Work out the finished part from the listing and answer in its coordinate system (mm). Face numbers are marked on the shaded views. A direction names the side the tool comes from. Round coordinates to 2 decimals unless told otherwise and drop trailing zeros. Order: outer loops, then holes, each group sorted by start corner. A loop starts at its lowest first (then second) coordinate and runs counter-clockwise, first axis right, second up. Notation, with made-up numbers: (80.25, 61) - (134.25, 61) arc R13 cw to (134.25, 81) - close; hole circle Ø9 at (87.25, 17.5). An arc over 180 degrees is marked (long way). One line per question, with ' | ' between items. Start each with the question number.
from build123d import *

# Parameters (mm, degrees)
BOSS_EXTRUDE1_DEPTH = 15.875
BOSS_EXTRUDE2_DEPTH = 3.175
CUT_EXTRUDE1_REACH  = 24.393
FILLET2_R           = 1.778
FILLET3_R           = 1.778


with BuildPart() as part:
    # Sketch1 → Boss-Extrude1 (new body)
    with BuildSketch(Plane(origin=(0, 0, 0), x_dir=(0, 0, -1), z_dir=(1, 0, 0))):
        Polygon((0, 0), (-1.016, 0), (-1.016, 10.541), (13.97, 10.541), (13.97, 0), (12.954, 0), (12.954, 9.525), (0, 9.525), align=None)
    extrude(amount=BOSS_EXTRUDE1_DEPTH)

    # Sketch2 → Boss-Extrude2 (add)
    with BuildSketch(Plane.XZ):
        with BuildLine():
            Line((9.525, 2.286), (9.525, 1.016))
            Line((9.525, 1.016), (0, 1.016))
            Line((0, 1.016), (0, 2.286))
            ThreePointArc((0, 2.286), (4.7625, 7.0485), (9.525, 2.286))
        make_face()
    boss_extrude2 = extrude(amount=-BOSS_EXTRUDE2_DEPTH)

    # Sketch4 → Cut-Extrude1 (cut, up to next)
    with BuildSketch(Plane(origin=(0, 3.175, 0), x_dir=(1, 0, 0), z_dir=(0, 1, 0)), mode=Mode.PRIVATE) as cut_extrude1_sk1:
        with BuildLine():
            Line((8.255, -2.286), (1.27, -2.286))
            ThreePointArc((1.27, -2.286), (4.7625, -5.7785), (8.255, -2.286))
        make_face()
    cut_extrude1_tool1 = extrude(cut_extrude1_sk1.sketch, amount=-CUT_EXTRUDE1_REACH, mode=Mode.PRIVATE) & part.part
    cut_extrude1 = cut_extrude1_tool1.solids().sort_by_distance((4.7625, 3.175, 3.768263))[0]
    add(cut_extrude1, mode=Mode.SUBTRACT)

    # Fillet2
    # the kernel refuses this fillet: 1.778 mm, written as the material it adds along each edge
    with BuildSketch(Plane(origin=(9.525, 3.175, 1.016), x_dir=(0, 1, 0), z_dir=(-1, 0, 0))) as fillet2_piece_1_section:
        with BuildLine():
            CenterArc((FILLET2_R, -FILLET2_R), FILLET2_R, 90, 90)
            Line((0, -FILLET2_R), (0, 0))
            Line((0, 0), (FILLET2_R, 0))
        make_face()
    fillet2_piece_1 = extrude(amount=9.525, mode=Mode.PRIVATE)
    fillet2_piece_1 = split(fillet2_piece_1, bisect_by=Plane(origin=(9.463917271, 3.688621556, 2.286), z_dir=(0, 0, -1)), keep=Keep.TOP, mode=Mode.PRIVATE)
    add(fillet2_piece_1)
    with BuildSketch(Plane(origin=(13.97, 3.175, 1.016), x_dir=(0, 1, 0), z_dir=(-1, 0, 0))) as fillet2_piece_2_section:
        with BuildLine():
            CenterArc((FILLET2_R, -FILLET2_R), FILLET2_R, 90, 90)
            Line((0, -FILLET2_R), (0, 0))
            Line((0, 0), (FILLET2_R, 0))
        make_face()
    fillet2_piece_2 = extrude(amount=18.415, mode=Mode.PRIVATE)
    fillet2_piece_2 = fillet2_piece_2 & Plane(origin=(4.7625, 3.197144068, 2.286), x_dir=(-1, 0, 0), z_dir=(0, -1, 0)) * Cylinder(4.7625, 44, mode=Mode.PRIVATE)
    fillet2_piece_2 = fillet2_piece_2 - Plane(origin=(4.7625, 3.197144068, 2.286), x_dir=(-1, 0, 0), z_dir=(0, 1, 0)) * Cylinder(3.4925, 44, mode=Mode.PRIVATE)
    add(fillet2_piece_2)

    # Mirror2: Boss-Extrude2 across plane
    add(boss_extrude2.mirror(Plane.XY.offset(-6.477)))

    # Mirror3: Cut-Extrude1 across plane
    add(cut_extrude1.mirror(Plane.XY.offset(-6.477)), mode=Mode.SUBTRACT)

    # Fillet3
    # the kernel refuses this fillet: 1.778 mm, written as the material it adds along each edge
    with BuildSketch(Plane(origin=(9.525, 3.175, -13.97), x_dir=(0, 0, -1), z_dir=(-1, 0, 0))) as fillet3_piece_1_section:
        with BuildLine():
            CenterArc((FILLET3_R, -FILLET3_R), FILLET3_R, 90, 90)
            Line((0, -FILLET3_R), (0, 0))
            Line((0, 0), (FILLET3_R, 0))
        make_face()
    fillet3_piece_1 = extrude(amount=9.525, mode=Mode.PRIVATE)
    fillet3_piece_1 = split(fillet3_piece_1, bisect_by=Plane(origin=(9.46391727, 3.688621585, -15.24), z_dir=(0, 0, 1)), keep=Keep.TOP, mode=Mode.PRIVATE)
    add(fillet3_piece_1)
    with BuildSketch(Plane(origin=(13.97, 3.175, -13.97), x_dir=(0, 0, -1), z_dir=(-1, 0, 0))) as fillet3_piece_2_section:
        with BuildLine():
            CenterArc((FILLET3_R, -FILLET3_R), FILLET3_R, 90, 90)
            Line((0, -FILLET3_R), (0, 0))
            Line((0, 0), (FILLET3_R, 0))
        make_face()
    fillet3_piece_2 = extrude(amount=18.415, mode=Mode.PRIVATE)
    fillet3_piece_2 = fillet3_piece_2 & Plane(origin=(4.7625, 3.197144068, -15.24), x_dir=(-1, 0, 0), z_dir=(0, -1, 0)) * Cylinder(4.7625, 44, mode=Mode.PRIVATE)
    fillet3_piece_2 = fillet3_piece_2 - Plane(origin=(4.7625, 3.197144068, -15.24), x_dir=(-1, 0, 0), z_dir=(0, 1, 0)) * Cylinder(3.4925, 44, mode=Mode.PRIVATE)
    add(fillet3_piece_2)


solid = part.part
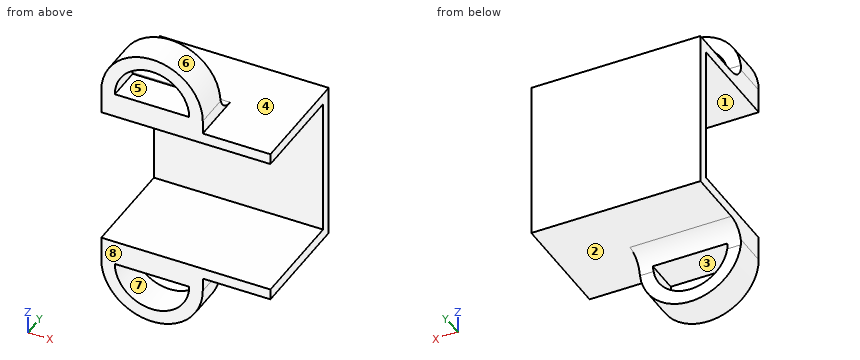
1) For the marked faces 1, 2, 3 and 4, determine the directions among +Z, -Z, +X, -X, +Y, -Y from which every point of the face is accessible in a straight line to the end or side of a thin tool.
2) Section D-D on x = 13.25 is taken. Give the vertices of the cut face in (y, z) (3 decimals), and give its area (3 significant figures).
3) Section C-C on x = 7 is taken. Give the vertices of the cut face in (y, z) (3 decimals).
4) Section A-A on y = 6 is taken. Give the vertices of the cut face in (x, z) (3 decimals).
5) Determine the mould class of the marked faces 5, 6, 7 and 8 for opening direction Z: released by +Z, released by -Z, zero draft, split by the parting line, or undercut.
6) Straight lines are drawn through the part: line 1 (Z direction, x = 13.75, y = 5); line 2 (Y direction, x = 4, z = -5.75) (3 decimals); line 3 (X direction, y = 2, z = 1.25) (3 decimals). For each, find the intervals that lie inside material, in ascending order.
7) Flat-ended cylindrical pins translate along their axes: pin 1 (0.6 mm diameter, centred on y = 3, z = -14.5, fed in from +X) (3 decimals); pin 2 (3 mm diameter, centred on x = 11.5, y = 5.5, fed in from -Z); pin 3 (3 mm diameter, centred on x = 2.5, z = 3, fed in from +Y). Find the tip coordinate at first contact, or state that the pin passes through.
Recorded:
1) face 1: +X, -X, -Y | face 2: -Z, +X, +Y | face 3: +Y, -Y | face 4: +Z, +X, +Y
2) outline: (0, -13.97) - (10.541, -13.97) - (10.541, 1.016) - (0, 1.016) - (0, 0) - (9.525, 0) - (9.525, -12.954) - (0, -12.954) - close | area: 34.6 mm²
3) outline: (0, -19.444) - (3.175, -19.444) - (3.175, -17.922) - (0, -17.922) - close; (0, -15.24) - (3.249, -15.24) arc R1.778 cw to (4.953, -13.97) - (10.541, -13.97) - (10.541, 1.016) - (4.953, 1.016) arc R1.778 cw to (3.249, 2.286) - (0, 2.286) - (0, 0) - (9.525, 0) - (9.525, -12.954) - (0, -12.954) - close; (0, 4.968) - (3.175, 4.968) - (3.175, 6.49) - (0, 6.49) - close
4) outline: (0, -13.97) - (15.875, -13.97) - (15.875, -12.954) - (0, -12.954) - close; (0, 0) - (15.875, 0) - (15.875, 1.016) - (0, 1.016) - close
5) face 5: undercut | face 6: released by +Z | face 7: undercut | face 8: zero draft
6) line 1: z = -13.97 to -12.95, 0 to 1.02 | line 2: y = 9.525 to 10.541 | line 3: x = 0 to 9.525
7) pin 1: stops at x = 9.525 | pin 2: stops at z = -13.97 | pin 3: stops at y = 3.73
